Autodesk Inventor part; units mm, degrees
ref_plane "YZ Plane" through (0, 0, 0) normal (1, 0, 0) x (0, 1, 0)
ref_plane "XZ Plane" through (0, 0, 0) normal (0, 1, 0) x (-1, 0, 0)
ref_plane "XY Plane" through (0, 0, 0) normal (0, 0, 1) x (1, 0, 0)
sketch "Sketch1" plane through (0, 0, 0) normal (0, 0, 1) x (1, 0, 0)
  line L0 (2448.8434, -559.2477) -> (2606.8434, -559.2477)
  line L1 (2606.8434, -489.2477) -> (2448.8434, -489.2477)
  line L2 (2448.8434, -489.2477) -> (2448.8434, -559.2477)
  circle A0 centre (2462.8434, -549.2477) radius 5
  arc A1 (2487.8434, -526.7477) -> (2487.8434, -521.7477) centre (2487.8434, -524.2477) ccw
  arc A2 (2487.8434, -521.7477) -> (2487.8434, -526.7477) centre (2487.8434, -524.2477) ccw
  line L3 (2487.3434, -526.7477) -> (2488.3434, -526.7477)
  line L4 (2488.3434, -521.7477) -> (2487.3434, -521.7477)
  circle A3 centre (2462.8434, -499.2477) radius 5
  line L5 (2606.8434, -559.2477) -> (2606.8434, -489.2477)
  circle A4 centre (2592.8434, -549.2477) radius 5
  circle A5 centre (2592.8434, -499.2477) radius 5
  circle A6 centre (2567.8434, -524.2477) radius 2.5
  point P0 (0, 0)
extrude "Extrusion1" add sketch "Sketch1" along normal blind 16
sketch "Sketch2" plane through (0, 0, 0) normal (0, 0, -1) x (-1, 0, 0)
  circle A0 centre (-2487.8434, -524.2477) radius 2.5
  circle A1 centre (-2567.8434, -524.2477) radius 2.5
  circle A2 centre (-2589.8434, -524.2477) radius 12.5
  circle A3 centre (-2465.8434, -524.2477) radius 12.5
  line L0 (-2527.8434, -524.2477) -> (-2527.8434, -513.4708)
  point P0 (0, 0)
  dimension "d2" = 25
  dimension "d3" = 25
  dimension "d8" = 124
  dimension "d9" = 62
extrude "Extrusion2" add sketch "Sketch2" along normal blind 177 contours A2 | A3
properties part number "ADSK-MH-10030" material "Aluminum 6061"
Read the model definition and answer for the solid it produces. Units are mm, in the model's axes. A direction names the side the tool comes from. Round coordinates to 2 decimals unless told otherwise and drop trailing zeros. Loops run counter-clockwise (first coordinate to the right, second up) from the corner with the lowest first, then second, coordinate; pieces in that order, holes last. Notation, with made-up numbers: (33.25, -12.75) - (86.25, -12.75) arc R21 ccw to (86.25, 26.25) - close; hole circle Ø5 at (40, -6.75). An arc over 180 degrees is marked (long way). One line per question, with ' | ' between items. Start each with the question number.
Q1. Section D-D on y = -518 is taken. Give the vertices of the cut face in (x, z), plus the area to 3 significant figures.
Q2. Section B-B on y = -534.5 is taken. Give the vertices of the cut face in (x, z), plus the area to 3 significant figures.
Q3. For a pull along Y with two mould halves and no side action, classify faces 1 (the flat face through (2466, -524, -177)), 2 (the cylindrical face through (2578.297, -519.46, -87.261)), 3 (the cylindrical face through (2467.613, -550.75, 7.888)) as +Y half, -Y half, draft (parallel to the pull), parting line (faces both ways), or undercut.
Q4. Section C-C on z = -118 is taken. Give the vertices of the cut face in (x, y), plus the area to 3 significant figures.
Q5. Find the intervals of material crossed by L1, parallel to Z at x = 2551, y = -499; L2, parallel to X at y = -532, z = -5; L3, parallel to X at y = -515, z = -167, in increasing order.
Q6. Section A-A on x = 2556 is taken. Give the vertices of the cut face in (y, z), plus the area to 3 significant figures.
Q7. Flat-ended cylindrical pins translate along their axes: pin 1 (3 mm diameter, centred on y = -514.5, z = -72, fed in from +X); pin 2 (11.5 mm diameter, centred on x = 2592.84, y = -549.25, fed in from -Z); pin 3 (10 mm diameter, centred on y = -540.5, z = -134, fed in from -X). Find the tip coordinate at first contact, or state that the pin passes through.
Q8. For faces 4 (the flat face through (2527, -559.248, 8)), 5 (the cylindrical face through (2454.297, -519.46, -87.261)), determine the directions among +Z, -Z, +X, -X, +Y, -Y from which every point of the face is accessible in a straight line to the end or side of a thin tool.
Established:
1) outline: (2448.84, 0) - (2455.02, 0) - (2455.02, -177) - (2476.67, -177) - (2476.67, 0) - (2579.02, 0) - (2579.02, -177) - (2600.67, -177) - (2600.67, 0) - (2606.84, 0) - (2606.84, 16) - (2448.84, 16) - close | area: 10,200 mm²
2) outline: (2448.84, 0) - (2458.69, 0) - (2458.69, -177) - (2472.99, -177) - (2472.99, 0) - (2582.69, 0) - (2582.69, -177) - (2596.99, -177) - (2596.99, 0) - (2606.84, 0) - (2606.84, 16) - (2448.84, 16) - close | area: 7,590 mm²
3) face 1: draft | face 2: parting line | face 3: undercut
4) outline: circle Ø25 at (2465.84, -524.25); circle Ø25 at (2589.84, -524.25) | area: 982 mm²
5) L1: 0 to 16 | L2: 2456.04 to 2475.65, 2580.04 to 2599.65 | L3: 2457.43 to 2474.25, 2581.43 to 2598.25
6) outline: (-559.25, 0) - (-489.25, 0) - (-489.25, 16) - (-559.25, 16) - close | area: 1,120 mm²
7) pin 1: x = 2599.24 | pin 2: z = 0 | pin 3: x = 2460.4
8) face 4: +Z, -Z, +X, -X, -Y | face 5: -Z
